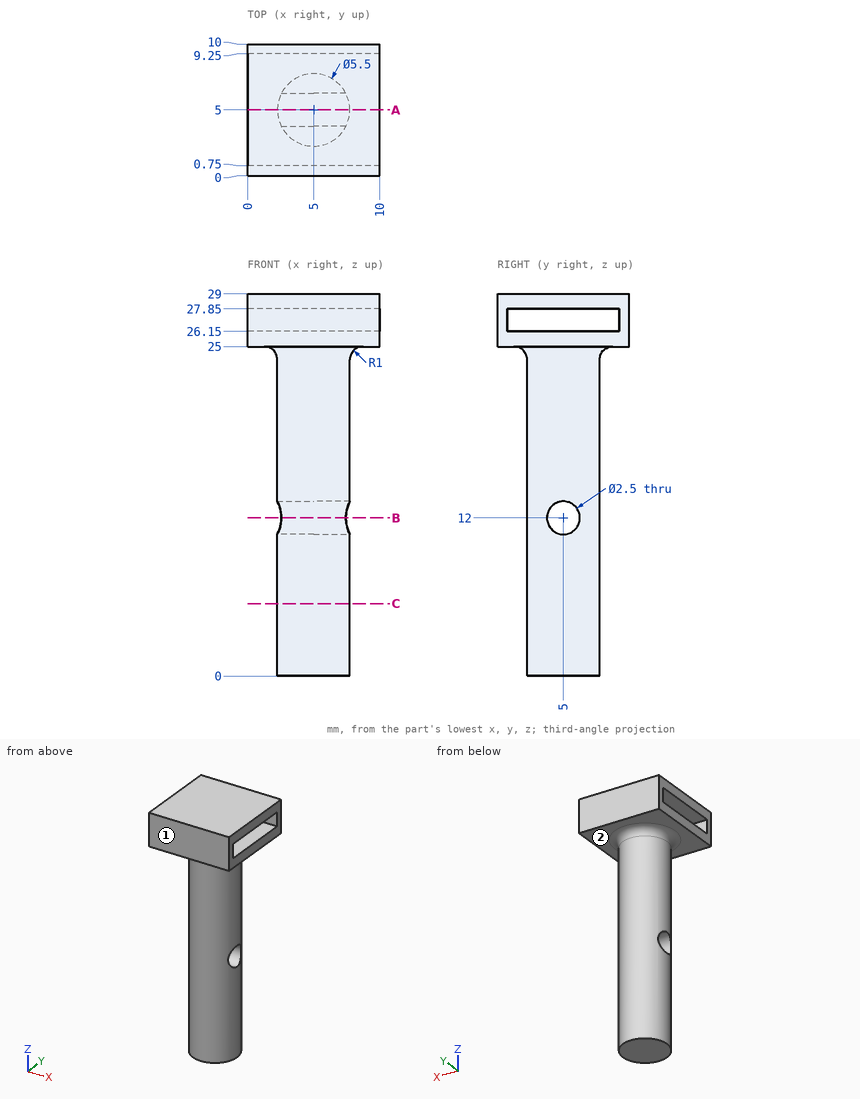
Design review of the part shown in the three views and the two pictorial views. Dimensions are in mm from the part's minimum x, y and z. A direction names the side the tool comes from. Coordinates: 2 decimals unless noted, no trailing zeros. Loops run counter-clockwise (first coordinate to the right, second up) from the corner with the lowest first, then second, coordinate; pieces in that order, holes last.
(1) Wall thickness on L1, parallel to Z at x = 4.05, y = 5; L2, parallel to Z at x = 5.5, y = 1.25: over which ranges is each line inside the solid? List them lowest first.
Determined:
L1: z = 0 to 10.75, 13.25 to 26.15, 27.85 to 29
L2: z = 25 to 26.15, 27.85 to 29
(2) Tool access review of the marked faces 1 and 2: name each direction out of +Z, -Z, +X, -X, +Y, -Y from which nothing blocks a thin tool from reaching the whole face with its end or side.
Determined:
face 1: +Z, -Z, +X, -X, -Y
face 2: -Z
(3) Consider section C-C, the plane z = 5.5. Give the boundary of the cut face in (x, y).
Determined:
outline: circle Ø5.5 at (5, 5)
(4) Consider section B-B, the plane z = 12. Give the boundary of the cut face in (x, y).
Determined:
outline: (2.55, 3.75) arc R2.75 ccw to (7.45, 3.75) - close; (2.55, 6.25) - (7.45, 6.25) arc R2.75 ccw to start
(5) Consider section A-A, the plane y = 5. Give the number of separate pieces and of enclosed holes in the cut face, plus the area to 3 significant figures.
Determined:
separate pieces: 3
enclosed holes: 0
area: 147 mm2
(6) Insertion check: P1, Ø1.5, axis at x = 7.5, y = 2, coming from the -Z side; P2, Ø2, axis at y = 3, z = 23, coming from the -X side; P3, Ø2, axis at y = 5, z = 12, coming from the +X side; P4, Ø3, axis at y = 1.5, z = 8.5, coming from the -X side. Each pin has a flat end and moves straight along its axis. Give the tip position at first contact, or say it passes through.
Determined:
P1: stops at z = 24.8
P2: stops at x = 2.44
P3: passes through
P4: stops at x = 3.11
